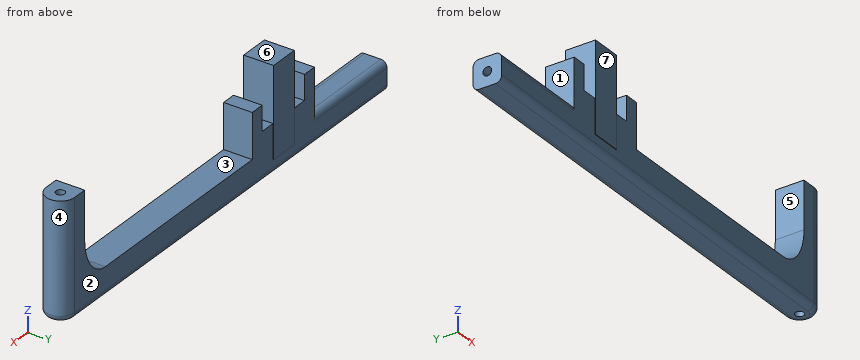
```python
from build123d import *

# Parameters (mm, degrees)
SKETCH_1_W           = 2.4
SKETCH_1_H           = 2.4
EXTRUDE_1_DEPTH      = 7.2
EXTRUDE_2_DEPTH      = 23
EXTRUDE_2_DEPTH_BACK = 12
SKETCH_4_W           = 2.3
SKETCH_4_H           = 2.3
EXTRUDE_3_DEPTH      = 7
EXTRUDE_3_DEPTH_BACK = 2.3
SKETCH_5_R           = 0.35
SKETCH_6_R           = 0.35
CUT_EXTRUDE_1_DEPTH  = 10
FILLET_1_SIZE        = 2.4
FILLET_1_SIZE_2      = 3.2
FILLET_2_R           = 0.5
EXTRUDE_START        = -1.5
SKETCH_7_W           = 1.15
SKETCH_7_H           = 0.5
SKETCH_7_H_2         = 1.3
SKETCH_7_H_3         = 2.3
EXTRUDE_4_DEPTH      = 5.1
SKETCH_8_W           = 7.2
SKETCH_8_H           = 2.3
EXTRUDE_5_DEPTH      = 3.1


with BuildPart() as part:
    # 草图1 → 凸台-拉伸1 (new body)
    with BuildSketch(Plane.XY):
        Rectangle(SKETCH_1_W, SKETCH_1_H)
    extrude(amount=EXTRUDE_1_DEPTH)

    # 草图4 → 凸台-拉伸2 (add, two sides: drawn at the far end of the back side and taken through both)
    with BuildSketch(Plane(origin=(0, 0, 0), x_dir=(0, 0, -1), z_dir=(1, 0, 0)).offset(-EXTRUDE_2_DEPTH_BACK)):
        Rectangle(SKETCH_4_W, SKETCH_4_H)
    extrude(amount=EXTRUDE_2_DEPTH + EXTRUDE_2_DEPTH_BACK)

    # 草图5 → 凸台-拉伸3 (add, two sides: drawn at the far end of the back side and taken through both)
    with BuildSketch(Plane.XY.offset(1.15).offset(-EXTRUDE_3_DEPTH_BACK)):
        with BuildLine():
            Line((23, 0), (23, 1.15))
            Line((23, 1.15), (24.15, 1.15))
            ThreePointArc((24.15, 1.15), (25.3, 0), (24.15, -1.15))
            Line((24.15, -1.15), (23, -1.15))
            Line((23, -1.15), (23, 0))
        make_face()
        with Locations(Location((24.15, 0, 0), (0, 0, 180))):
            Circle(SKETCH_5_R, mode=Mode.SUBTRACT)
    extrude(amount=EXTRUDE_3_DEPTH + EXTRUDE_3_DEPTH_BACK)

    # 草图6 → 切除-拉伸1 (cut)
    with BuildSketch(Plane.ZY.offset(12)):
        Circle(SKETCH_6_R)
    extrude(amount=-CUT_EXTRUDE_1_DEPTH, mode=Mode.SUBTRACT)

    # 圆角1
    # an asymmetric fillet: 3.2, 2.4 mm, written as the material it adds along each edge
    with BuildSketch(Plane(origin=(23, 1.15, 1.15), x_dir=(-1, 0, 0), z_dir=(0, -1, 0))) as fillet_1_piece_1:
        with BuildLine():
            Bezier((FILLET_1_SIZE, 0), (0, 0), (0, -FILLET_1_SIZE_2), weights=[1, 0.707106781, 1])
            Line((0, -FILLET_1_SIZE_2), (0, 0))
            Line((0, 0), (FILLET_1_SIZE, 0))
        make_face()
    extrude(amount=2.3)

    # 圆角2
    fillet_2_edges = [part.edges().sort_by_distance(p)[0] for p in [
        (-6.6, -1.15, 1.15),
        (6.075, -1.15, -1.15),
        (-6.6, 1.15, 1.15),
        (6.075, 1.15, -1.15),
        (25.3, 0, -1.15),
    ]]
    fillet(fillet_2_edges, radius=FILLET_2_R)

    # 草图7 → 凸台-拉伸4 (add)
    with BuildSketch(Plane.XY.offset(1.15).offset(EXTRUDE_START)):
        with Locations((-3.025, 0.9)):
            Rectangle(SKETCH_7_W, SKETCH_7_H)
        with Locations((-3.025, 0)):
            Rectangle(SKETCH_7_W, SKETCH_7_H_2)
        with Locations((-3.025, -0.9)):
            Rectangle(SKETCH_7_W, SKETCH_7_H)
        with Locations((3.025, 0)):
            Rectangle(SKETCH_7_W, SKETCH_7_H_3)
    extrude(amount=EXTRUDE_4_DEPTH)

    # 草图8 → 凸台-拉伸5 (add)
    with BuildSketch(Plane.XY.offset(1.15).offset(EXTRUDE_START)):
        Rectangle(SKETCH_8_W, SKETCH_8_H)
    extrude(amount=EXTRUDE_5_DEPTH)


solid = part.part
```
The model under review builds one solid part; all positions refer to its coordinate system, in mm. Face numbers are marked on the shaded views. A direction names the side the tool comes from. Round coordinates to 2 decimals unless told otherwise and drop trailing zeros. Write each loop counter-clockwise with the first axis right and the second up, starting at its lowest first coordinate (ties: lowest second). Pieces come first, ordered by that corner, then holes. Notation, with made-up numbers: M -14,18 L 32,18 A21 ccw 32,34 Z; hole C 58,40.25 d4. An arc over 180 degrees is marked long. Use CSV: the item, a comma, the result in double quotes. Start each with the question number.
(1) For line 1 along Y through (x, z) = (-9.5, 0); line 2 along X through (y, z) = (-0.95, 3.5); line 3 along X through (y, z) = (-1, 3), list the stretches that pass through material, from the lowest coordinate up.
(2) We need section D-D, the plane z = 3.5. State how many separate pieces and enclosed holes the cut face has, then the cut area to 3 significant figures.
(3) The part is to be moulded in two halves that separate along X. For the marked faces 1, 2, 3 and 4, say which applies: +X half, -X half, draft (parallel to the pull), parting line (faces both ways), or undercut.
(4) We need section A-A, the plane z = 6.25. State the section outline as (x, y) points.
(5) We need section C-C, the plane x = 5. State the section outline as (y, z) points, then the cut area to 3 significant figures.
(6) Tool access review of the marked faces 5, 6 and 7: name each direction out of +Z, -Z, +X, -X, +Y, -Y from which nothing blocks a thin tool from reaching the whole face with its end or side.
(7) Clearance check with flat-ended pins moving along their axes: P1, Ø1, axis at x = -7, y = 0, coming from the +Z side; P2, Ø0.6, axis at x = 3, y = -0.5, coming from the +Z side; P3, Ø0.6, axis at x = -2, y = 0, coming from the +Z side. State where each tip first meets the part, or that it passes through.
(8) We need section B-B, the plane z = 7.75. State the section outline as (x, y) points, then the cut area to 3 significant figures.
Findings:
1,line 1,"-1.15 to -0.35, 0.35 to 1.15"
1,line 2,"-3.6 to -2.45, -1.2 to 1.2, 2.45 to 3.6, 22.91 to 24.8"
1,line 3,"-3.6 to -2.45, -1.2 to 1.2, 2.45 to 3.6, 22.78 to 24.72"
2,separate pieces,"4"
2,enclosed holes,"1"
2,area,"15.6 mm^2"
3,face 1,"-X half"
3,face 2,"draft"
3,face 3,"undercut"
3,face 4,"+X half"
4,outline,"M -1.2,-1.2 L 1.2,-1.2 L 1.2,1.2 L -1.2,1.2 Z; M 23,-1.15 L 24.15,-1.15 A1.15 ccw 24.15,1.15 L 23,1.15 Z; hole C 24.15,0 d0.7"
5,outline,"M -1.15,-0.65 A0.5 ccw -0.65,-1.15 L 0.65,-1.15 A0.5 ccw 1.15,-0.65 L 1.15,1.15 L -1.15,1.15 Z"
5,area,"5.18 mm^2"
6,face 5,"+Z, +Y, -Y"
6,face 6,"+Z, -X, +Y, -Y"
6,face 7,"+Z, -Z, +X, -X, -Y"
7,P1,"z = 1.15"
7,P2,"z = 4.75"
7,P3,"z = 2.75"
8,outline,"M 23,-1.15 L 24.15,-1.15 A1.15 ccw 24.15,1.15 L 23,1.15 Z; hole C 24.15,0 d0.7"
8,area,"4.34 mm^2"
